from build123d import *

# Parameters (mm, degrees)
BOSS_EXTRUDE1_DEPTH   = 3.81
LPATTERN1_COUNT       = 2
LPATTERN1_PITCH       = 60.94
LPATTERN2_COUNT       = 2
LPATTERN2_PITCH       = 85.06
LPATTERN3_COUNT       = 2
LPATTERN3_PITCH       = 60.94
LPATTERN5_COUNT       = 2
LPATTERN5_PITCH       = 85.06
LPATTERN6_COUNT       = 2
LPATTERN6_PITCH       = 60.94
BODY_MOVE_COPY1_ANGLE = 180
BODY_MOVE_COPY2_ANGLE = 120
BODY_MOVE_COPY3_ANGLE = 120
SKETCH2_R             = 9.5
BOSS_EXTRUDE2_DEPTH   = 228.49


with BuildPart() as part:
    # Sketch1 → Boss-Extrude1 (new, symmetric)
    with BuildSketch(Plane.XY):
        with BuildLine():
            Line((5.499261314, 15.875), (10.998522628, 6.35))
            ThreePointArc((10.998522628, 6.35), (0, -12.7), (-10.998522628, 6.35))
            Line((-10.998522628, 6.35), (-5.499261314, 15.875))
            ThreePointArc((-5.499261314, 15.875), (0, 19.05), (5.499261314, 15.875))
        make_face()
    extrude(amount=BOSS_EXTRUDE1_DEPTH, both=True)


with BuildPart() as lpattern1_1:
    # LPattern1: pattern copy
    add(part.part.moved(Location(Vector(0, 0, 1) * (1 * LPATTERN1_PITCH))))


with BuildPart() as lpattern2_1:
    # LPattern2: pattern copy
    add(lpattern1_1.part.moved(Location(Vector(0, 0, 1) * (1 * LPATTERN2_PITCH))))


with BuildPart() as lpattern3_1:
    # LPattern3: pattern copy
    add(lpattern2_1.part.moved(Location(Vector(0, 0, 1) * (1 * LPATTERN3_PITCH))))


with BuildPart() as lpattern5_1:
    # LPattern5: pattern copy
    add(lpattern3_1.part.moved(Location(Vector(0, 0, 1) * (1 * LPATTERN5_PITCH))))


with BuildPart() as lpattern6_1:
    # LPattern6: pattern copy
    add(lpattern5_1.part.moved(Location(Vector(0, 0, 1) * (1 * LPATTERN6_PITCH))))


with BuildPart() as lpattern5_1_1:
    # Body-Move_Copy1: moved
    add(lpattern5_1.part.rotate(Axis((0, 0, 0), (0, 0, 1)), BODY_MOVE_COPY1_ANGLE))


with BuildPart() as lpattern2_1_1:
    # Body-Move_Copy1: moved
    add(lpattern2_1.part.rotate(Axis((0, 0, 0), (0, 0, 1)), BODY_MOVE_COPY1_ANGLE))


with BuildPart() as part_1:
    # Body-Move_Copy1: moved
    add(part.part.rotate(Axis((0, 0, 0), (0, 0, 1)), BODY_MOVE_COPY1_ANGLE))


with BuildPart() as lpattern3_1_1:
    # Body-Move_Copy2: moved
    add(lpattern3_1.part.rotate(Axis((0, 0, 0), (0, 0, -1)), BODY_MOVE_COPY2_ANGLE))


with BuildPart() as lpattern2_1_2:
    # Body-Move_Copy2: moved
    add(lpattern2_1_1.part.rotate(Axis((0, 0, 0), (0, 0, -1)), BODY_MOVE_COPY2_ANGLE))


with BuildPart() as lpattern1_1_1:
    # Body-Move_Copy3: moved
    add(lpattern1_1.part.rotate(Axis((0, 0, 0), (0, 0, 1)), BODY_MOVE_COPY3_ANGLE))


with BuildPart() as part_2:
    # Body-Move_Copy3: moved
    add(part_1.part.rotate(Axis((0, 0, 0), (0, 0, 1)), BODY_MOVE_COPY3_ANGLE))


    add(lpattern1_1_1.part)  # Boss-Extrude2 merges LPattern1_1

    add(lpattern2_1_2.part)  # Boss-Extrude2 merges LPattern2_1

    add(lpattern3_1_1.part)  # Boss-Extrude2 merges LPattern3_1

    add(lpattern5_1_1.part)  # Boss-Extrude2 merges LPattern5_1

    add(lpattern6_1.part)  # Boss-Extrude2 merges LPattern6_1
    # Sketch2 → Boss-Extrude2 (add, symmetric)
    with BuildSketch(Plane(origin=(0, 0, 176.47), x_dir=(-1, 0, 0), z_dir=(0, 0, -1))):
        with Locations(Location((0, 0, 0), (0, 0, 180))):
            Circle(SKETCH2_R)
    extrude(amount=BOSS_EXTRUDE2_DEPTH, both=True)


solid = part_2.part
CAD build for the part. Positions are in the model's coordinates, mm. A direction names the side the tool comes from. Give positions to 0.01 mm unless a question says otherwise; leave off trailing zeros. Write each loop counter-clockwise with the first axis right and the second up, starting at its lowest first coordinate (ties: lowest second). Pieces come first, ordered by that corner, then holes. Notation, with made-up numbers: (1.5, 66) - (53.5, 66) arc R30 ccw to (53.5, 92) - close; hole circle Ø7 at (52.25, 37.5). An arc over 180 degrees is marked (long way). Put each result on its own line as item: value.
(1) Drop flat-ended pins along their axis: pin 1 Ø12 at (x, z) = (4, 14.5) entering from -Y; pin 2 Ø10 at (x, z) = (11, 13.5) entering from -Y; pin 3 Ø2 at (y, z) = (6, 260.5) entering from -X. Give the stop position or say it passes through.
Working result:
pin 1: y = -9.5
pin 2: y = -7.37
pin 3: x = -8.08
(2) Wall check: L1, parallel to Z at x = 10, y = -7; L2, parallel to Z at x = -13.5, y = 11.5; L3, parallel to Z at x = -13, y = -10.5. Give the ranges that are in metal, low to high.
Working result:
L1: -3.81 to 3.81, 57.13 to 64.75, 142.19 to 149.81, 203.13 to 210.75, 288.19 to 295.81, 349.13 to 356.75
L2: 142.19 to 149.81
L3: 57.13 to 64.75
(3) Saw through at A-A (z = 299.5). List the corners of the cut face in (x, y).
Working result:
outline: circle Ø19 at (0, 0)
(4) Tool access for faces 4 (the flat face through (13.8, -1.5, 0.1)), 5 (the flat face through (-6, 12.7, 146)), 6 (the flat face through (-9, 4, 142.19)), 7 (the flat face through (8.287, -11.046, 292.053)): list every direction of +Z, -Z, +X, -X, +Y, -Y with a clear straight run to the whole face (end or side of a thin tool).
Working result:
face 4: -Z, +X, -Y
face 5: -Z, +X, -X, +Y
face 6: none
face 7: +Z, +X, -Y
(5) Pull direction Z, two halves, no side cores. Call faces 1 (the flat face through (7, 7, -3.81)), 2 (the cylindrical face through (-2.059, 9.274, 248.928)), 3 (the cylindrical face through (-2.059, 9.274, 380.518)): released by +Z, released by -Z, zero draft, split by the parting line, or undercut.
Working result:
face 1: released by -Z
face 2: undercut
face 3: zero draft
